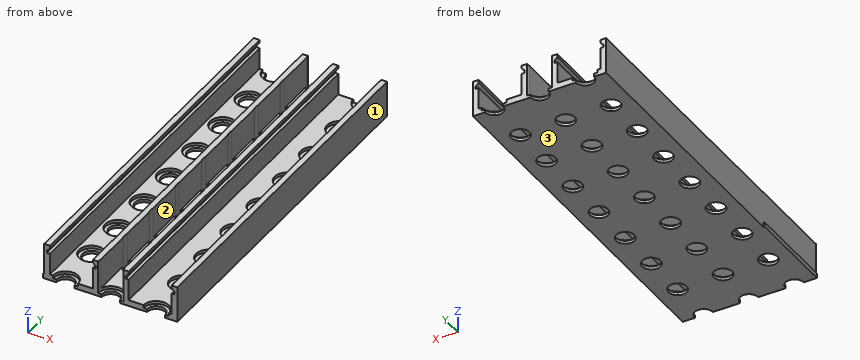
from build123d import *

# Parameters (mm, degrees)
PAD004_DEPTH            = 120
SKETCH016_W             = 44
SKETCH016_H             = 120
PAD005_DEPTH            = 2
LINEARPATTERN002_COUNT  = 2
LINEARPATTERN002_PITCH  = 26
SKETCH018_R             = 4.15
POCKET_DEPTH            = 1
POCKET_DEPTH_BACK       = 10
SKETCH017_R             = 3
POCKET004_DEPTH         = 2
LINEARPATTERN_COUNT     = 2
LINEARPATTERN_PITCH     = 15
SKETCH_W                = 1.5
SKETCH_H                = 30
PAD_DEPTH               = 0.4
BODY002_PLACEMENT_ANGLE = 180


with BuildPart() as part:
    # Sketch015 → Pad004 (new body)
    with BuildSketch(Plane(origin=(0.5, 0, 0), x_dir=(1, 0, 0), z_dir=(0, -1, 0))):
        Polygon((9, -6), (9, 6), (7.1, 6), (7.1, 5), (8.1, 4), (8.1, 3.2), (7.1, 3.2), (7.1, -4), (-7.1, -4), (-7.1, 3.2), (-8.1, 3.2), (-8.1, 4), (-7.1, 5), (-7.1, 6), (-9, 6), (-9, -6), align=None)
    pad004 = extrude(amount=PAD004_DEPTH)

    # Sketch016 (on DatumPlane) → Pad005 (join)
    with BuildSketch(Plane(origin=(-2, 0, -6), x_dir=(1, 0, 0), z_dir=(0, 0, 1))):
        with Locations((15.5, -60)):
            Rectangle(SKETCH016_W, SKETCH016_H)
    extrude(amount=PAD005_DEPTH)

    # LinearPattern002: Pad004 ×2
    with Locations(*[(i * LINEARPATTERN002_PITCH, 0, 0) for i in range(1, LINEARPATTERN002_COUNT)]):
        add(pad004)

    # Sketch018 → Pocket (cut, two sides)
    with BuildSketch(Plane(origin=(-16.5, -215.5, -4), x_dir=(1, 0, 0), z_dir=(0, 0, 1))) as pocket_sk:
        with Locations((15, 95.5)):
            Circle(SKETCH018_R)
        with Locations((45, 95.5)):
            Circle(SKETCH018_R)
        with Locations((30, 110.5)):
            Circle(SKETCH018_R)
        with Locations((60, 110.5)):
            Circle(SKETCH018_R)
        with Locations((90, 110.5)):
            Circle(SKETCH018_R)
        with Locations((15, 125.5)):
            Circle(SKETCH018_R)
        with Locations((45, 125.5)):
            Circle(SKETCH018_R)
        with Locations((75, 125.5)):
            Circle(SKETCH018_R)
        with Locations((105, 125.5)):
            Circle(SKETCH018_R)
        with Locations((15, 155.5)):
            Circle(SKETCH018_R)
        with Locations((45, 155.5)):
            Circle(SKETCH018_R)
        with Locations((75, 155.5)):
            Circle(SKETCH018_R)
        with Locations((60, 140.5)):
            Circle(SKETCH018_R)
        with Locations((30, 140.5)):
            Circle(SKETCH018_R)
        with Locations((90, 140.5)):
            Circle(SKETCH018_R)
        with Locations((105, 155.5)):
            Circle(SKETCH018_R)
        with Locations((30, 170.5)):
            Circle(SKETCH018_R)
        with Locations((60, 170.5)):
            Circle(SKETCH018_R)
        with Locations((90, 170.5)):
            Circle(SKETCH018_R)
        with Locations((15, 185.5)):
            Circle(SKETCH018_R)
        with Locations((45, 185.5)):
            Circle(SKETCH018_R)
        with Locations((75, 185.5)):
            Circle(SKETCH018_R)
        with Locations((105, 185.5)):
            Circle(SKETCH018_R)
        with Locations((30, 200.5)):
            Circle(SKETCH018_R)
        with Locations((60, 200.5)):
            Circle(SKETCH018_R)
        with Locations((90, 200.5)):
            Circle(SKETCH018_R)
        with Locations((15, 215.5)):
            Circle(SKETCH018_R)
        with Locations((45, 215.5)):
            Circle(SKETCH018_R)
        with Locations((120, 110.5)):
            Circle(SKETCH018_R)
        with Locations((120, 140.5)):
            Circle(SKETCH018_R)
        with Locations((120, 170.5)):
            Circle(SKETCH018_R)
        with Locations((120, 200.5)):
            Circle(SKETCH018_R)
        with Locations((0, 110.5)):
            Circle(SKETCH018_R)
        with Locations((0, 140.5)):
            Circle(SKETCH018_R)
        with Locations((0, 170.5)):
            Circle(SKETCH018_R)
        with Locations((0, 200.5)):
            Circle(SKETCH018_R)
    pocket = extrude(amount=-POCKET_DEPTH, mode=Mode.SUBTRACT) + extrude(pocket_sk.sketch, amount=POCKET_DEPTH_BACK, mode=Mode.SUBTRACT)

    # Sketch017 → Pocket004 (cut)
    with BuildSketch(Plane(origin=(-16.5, -215.5, -4), x_dir=(1, 0, 0), z_dir=(0, 0, 1))):
        with Locations((15, 95.5)):
            Circle(SKETCH017_R)
        with Locations((45, 95.5)):
            Circle(SKETCH017_R)
        with Locations((30, 110.5)):
            Circle(SKETCH017_R)
        with Locations((60, 110.5)):
            Circle(SKETCH017_R)
        with Locations((90, 110.5)):
            Circle(SKETCH017_R)
        with Locations((15, 125.5)):
            Circle(SKETCH017_R)
        with Locations((45, 125.5)):
            Circle(SKETCH017_R)
        with Locations((75, 125.5)):
            Circle(SKETCH017_R)
        with Locations((105, 125.5)):
            Circle(SKETCH017_R)
        with Locations((15, 155.5)):
            Circle(SKETCH017_R)
        with Locations((45, 155.5)):
            Circle(SKETCH017_R)
        with Locations((75, 155.5)):
            Circle(SKETCH017_R)
        with Locations((60, 140.5)):
            Circle(SKETCH017_R)
        with Locations((30, 140.5)):
            Circle(SKETCH017_R)
        with Locations((90, 140.5)):
            Circle(SKETCH017_R)
        with Locations((105, 155.5)):
            Circle(SKETCH017_R)
        with Locations((30, 170.5)):
            Circle(SKETCH017_R)
        with Locations((60, 170.5)):
            Circle(SKETCH017_R)
        with Locations((90, 170.5)):
            Circle(SKETCH017_R)
        with Locations((15, 185.5)):
            Circle(SKETCH017_R)
        with Locations((45, 185.5)):
            Circle(SKETCH017_R)
        with Locations((75, 185.5)):
            Circle(SKETCH017_R)
        with Locations((105, 185.5)):
            Circle(SKETCH017_R)
        with Locations((30, 200.5)):
            Circle(SKETCH017_R)
        with Locations((60, 200.5)):
            Circle(SKETCH017_R)
        with Locations((90, 200.5)):
            Circle(SKETCH017_R)
        with Locations((15, 215.5)):
            Circle(SKETCH017_R)
        with Locations((45, 215.5)):
            Circle(SKETCH017_R)
        with Locations((120, 110.5)):
            Circle(SKETCH017_R)
        with Locations((120, 140.5)):
            Circle(SKETCH017_R)
        with Locations((120, 170.5)):
            Circle(SKETCH017_R)
        with Locations((120, 200.5)):
            Circle(SKETCH017_R)
        with Locations((0, 110.5)):
            Circle(SKETCH017_R)
        with Locations((0, 140.5)):
            Circle(SKETCH017_R)
        with Locations((0, 170.5)):
            Circle(SKETCH017_R)
        with Locations((0, 200.5)):
            Circle(SKETCH017_R)
    pocket004 = extrude(amount=-POCKET004_DEPTH, mode=Mode.SUBTRACT)

    # LinearPattern: Pocket004, Pocket ×2
    with Locations(*[(i * LINEARPATTERN_PITCH, 0, 0) for i in range(1, LINEARPATTERN_COUNT)]):
        add(pocket004, mode=Mode.SUBTRACT)
        add(pocket, mode=Mode.SUBTRACT)

    # Sketch (on Face79 of LinearPattern) → Pad (join)
    with BuildSketch(Plane(origin=(35.5, 0, 0), x_dir=(0, 0, 1), z_dir=(1, 0, 0))):
        with Locations((-5.25, 15)):
            Rectangle(SKETCH_W, SKETCH_H)
    extrude(amount=PAD_DEPTH)


with BuildPart() as part_1:
    # Body002 placement: moved
    add(part.part.moved(Location((2.5, -156, 9))).rotate(Axis((2.5, -156, 9), (0, 0, 1)), BODY002_PLACEMENT_ANGLE))


solid = part_1.part
Source: CAD feature listing. Evaluate the final solid. Frame: model axes, mm. Face numbers are marked on the shaded views. Round coordinates to 2 decimals unless told otherwise and drop trailing zeros. Return JSON: item names as keys, results as strings. Group by question number.
1. Section query B-B on x = -26. State how many separate pieces and enclosed holes the cut face has, and give its area (3 significant figures).
2. Mould query, pull axis X, two halves, no side actions, for the marked faces 1, 2 and 3. Classes: released by +X, released by -X, zero draft, split by the parting line, or undercut.
3. Pin query (flat end, axial travel): pin 1 (1.1 mm diameter, centred on y = -123, z = 14.5, fed in from -X); pin 2 (5.5 mm diameter, centred on x = -11, y = -141, fed in from +Z); pin 3 (4 mm diameter, centred on x = -10, y = -139.5, fed in from +Z); pin 4 (4 mm diameter, centred on x = -11.5, y = -46.5, fed in from +Z). Return the tip coordinate at first contact, or that it passes through.
4. Material intervals for line 1 along X through (y, z) = (-98, 10); line 2 along X through (y, z) = (-51, 10); line 3 along Z through (x, y) = (-30, -66), sorted ascending. Write a range as from..to.
Checks:
{
 "1": {"separate pieces": "8", "enclosed holes": "0", "area": "126 mm²"},
 "2": {"face 1": "released by +X", "face 2": "undercut", "face 3": "zero draft"},
 "3": {"pin 1": "stops at x = -33", "pin 2": "passes through", "pin 3": "stops at z = 4", "pin 4": "stops at z = 5"},
 "4": {"line 1": "x = -33..-31.1, -16.9..-15, -7..-5.1, 9.1..11", "line 2": "x = -33..-31.1, -16.9..-15.15, -6.85..-5.1, 9.1..11", "line 3": "z = 3..4"}
}
